For this review, take the finished solid that the model builds, in its own axes (mm). Coordinates: 2 decimals unless noted, no trailing zeros. Write each loop counter-clockwise with the first axis right and the second up, starting at its lowest first coordinate (ties: lowest second). Pieces come first, ordered by that corner, then holes. Notation, with made-up numbers: (-16.75, -34.5) -> (41.25, -34.5) arc R16 cw to (41.25, -22.5) -> close; hole circle Ø9 at (-34, 11). An arc over 180 degrees is marked (long way). Put each result on its own line as item: value. Start each with the question number.
Item 1: Consider section A-A on x = -60. Give the boundary of the cut face in (y, z).
Item 2: Consider section C-C on x = -90. Give the boundary of the cut face in (y, z), and give its area (3 significant figures).
Item 3: Insertion check: P1, Ø4.5, axis at x = -45, y = -25.98, coming from the +Z side; P2, Ø4, axis at x = -70.5, z = 4.5, coming from the +Y side; P3, Ø3, axis at x = -86, z = 5, coming from the +Y side; P4, Ø3, axis at y = 30, z = 6, coming from the +X side. Each pin has a flat end and moves straight along its axis. Give the tip position at first contact, or say it passes through.
Item 4: Consider section B-B on y = 1.5. Give the boundary of the cut face in (x, z).
Item 5: Consider section D-D on z = 2.75. Give the number of separate pieces and of enclosed holes in the cut face, and give its area (3 significant figures).
Item 6: To check wall thickness, follow L1, parallel to Y at x = -60, z = 4; L2, parallel to Y at x = -77, z = 5.5; L3, parallel to X at y = -28, z = 4. State the ranges of each line that lie inside material, in increasing order.
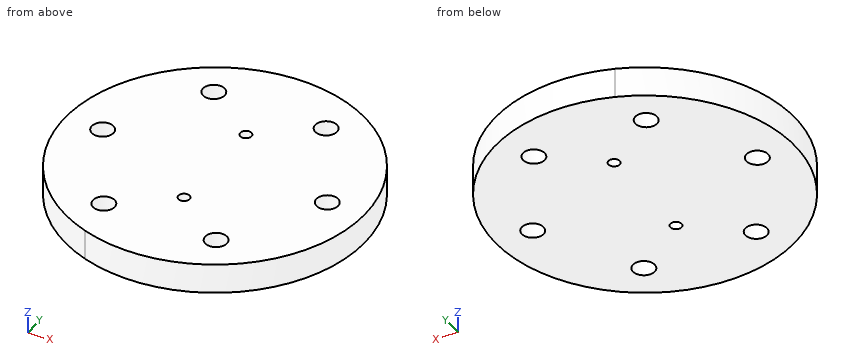
```python
from build123d import *

# Parameters (mm, degrees)
BOSS_EXTRU_1_DEPTH       = 8
ENL_V_START              = -10
ESQUISSE2_R              = 120
ENL_V_MAT_EXTRU_1_DEPTH  = 10
D_GAGEMENT_M51_OUTLINE_R = 2.9
D_GAGEMENT_M51_DEPTH     = 8
ESQUISSE5_R              = 1.5
ENL_V_MAT_EXTRU_2_DEPTH  = 10


# Read off the part's stored shape, not the designer's step: Dégagement M51
with BuildPart() as part:
    # Esquisse1 → Boss.-Extru.1 (new body)
    with BuildSketch(Plane.XY):
        with BuildLine():
            Line((-20, 56.568542495), (-73.333333333, 37.712361663))
            ThreePointArc((-73.333333333, 37.712361663), (-100, 0), (-73.333333333, -37.712361663))
            Line((-73.333333333, -37.712361663), (-20, -56.568542495))
            ThreePointArc((-20, -56.568542495), (34.641016151, -48.989794856), (60, 0))
            ThreePointArc((60, 0), (34.641016151, 48.989794856), (-20, 56.568542495))
        make_face()
    extrude(amount=BOSS_EXTRU_1_DEPTH)

    # Esquisse2 → Enlèv. mat.-Extru.1 (cut)
    with BuildSketch(Plane.XY.offset(8).offset(ENL_V_START)):
        with Locations((-60, 0)):
            Circle(ESQUISSE2_R)
        with BuildLine():
            ThreePointArc((-73.333333333, 37.712361663), (-100, 0), (-73.333333333, -37.712361663))
            ThreePointArc((-73.333333333, -37.712361663), (-20, 0), (-73.333333333, 37.712361663))
        make_face(mode=Mode.SUBTRACT)
    extrude(amount=ENL_V_MAT_EXTRU_1_DEPTH, mode=Mode.SUBTRACT)

    # Dégagement M51 outline → Dégagement M51 (cut)
    with BuildSketch(Plane.XY):
        with Locations((-90, 0)):
            Circle(D_GAGEMENT_M51_OUTLINE_R)
        with Locations((-75, -25.980762114)):
            Circle(D_GAGEMENT_M51_OUTLINE_R)
        with Locations((-45, -25.980762114)):
            Circle(D_GAGEMENT_M51_OUTLINE_R)
        with Locations((-30, 0)):
            Circle(D_GAGEMENT_M51_OUTLINE_R)
        with Locations((-45, 25.980762114)):
            Circle(D_GAGEMENT_M51_OUTLINE_R)
        with Locations((-75, 25.980762114)):
            Circle(D_GAGEMENT_M51_OUTLINE_R)
    extrude(amount=D_GAGEMENT_M51_DEPTH, mode=Mode.SUBTRACT)

    # Esquisse5 → Enlèv. mat.-Extru.2 (cut)
    with BuildSketch(Plane(origin=(819.686269666, 1346.410161514, 0), x_dir=(0, -1, 0), z_dir=(0, 0, -1))):
        with Locations(Location((1331.784714909, 879.686269666, 0), (0, 0, 90))):
            Circle(ESQUISSE5_R)
        with Locations(Location((1361.034715705, 879.686269666, 0), (0, 0, 90))):
            Circle(ESQUISSE5_R)
    extrude(amount=-ENL_V_MAT_EXTRU_2_DEPTH, mode=Mode.SUBTRACT)


solid = part.part
```
Return value:
1. outline: (-40, 0) -> (-16.12, 0) -> (-16.12, 8) -> (-40, 8) -> close; (-13.12, 0) -> (13.13, 0) -> (13.13, 8) -> (-13.12, 8) -> close; (16.13, 0) -> (40, 0) -> (40, 8) -> (16.13, 8) -> close
2. outline: (-26.46, 0) -> (-2.9, 0) -> (-2.9, 8) -> (-26.46, 8) -> close; (2.9, 0) -> (26.46, 0) -> (26.46, 8) -> (2.9, 8) -> close
2. area: 377 mm^2
3. P1: through
3. P2: y = 39.09
3. P3: y = 31.62
3. P4: x = -31.93
4. outline: (-99.97, 0) -> (-92.48, 0) -> (-92.48, 8) -> (-99.97, 8) -> close; (-87.52, 0) -> (-32.48, 0) -> (-32.48, 8) -> (-87.52, 8) -> close; (-27.52, 0) -> (-20.03, 0) -> (-20.03, 8) -> (-27.52, 8) -> close
5. separate pieces: 1
5. enclosed holes: 8
5. area: 4,850 mm^2
6. L1: -40 to -16.12, -13.12 to 13.13, 16.13 to 40
6. L2: -36.21 to -28.08, -23.88 to 23.88, 28.08 to 36.21
6. L3: -88.57 to -77.08, -72.92 to -47.08, -42.92 to -31.43
